from build123d import *

# Parameters (mm, degrees)
SKETCH_CAMERA_SEAT_W     = 16
SKETCH_CAMERA_SEAT_H     = 38
CAMERA_SEAT_DEPTH        = 3
FRONT_LIP_START          = 3
SKETCH_FRONT_LIP_W       = 16
SKETCH_FRONT_LIP_H       = 2.3
FRONT_LIP_DEPTH          = 7
REAR_LIP_START           = 3
SKETCH_REAR_LIP_W        = 16
SKETCH_REAR_LIP_H        = 2.3
REAR_LIP_DEPTH           = 4
STRAP_SLOTS_START        = -1
SKETCH_STRAP_SLOTS_W     = 8
SKETCH_STRAP_SLOTS_H     = 2.5
STRAP_SLOTS_DEPTH        = 5
M3_THROUGH_START         = -1
SKETCH_M3_THROUGH_R      = 1.7
M3_THROUGH_DEPTH         = 5
FLAT_HEAD_90DEG_START    = 1.5
SKETCH_FLAT_HEAD_90DEG_R = 1.5
FLAT_HEAD_90DEG_DEPTH    = 1.5
FLAT_HEAD_90DEG_TAPER    = -45


with BuildPart() as part:
    # Sketch_Camera_seat → Camera_seat (new body)
    with BuildSketch(Plane.XY):
        Rectangle(SKETCH_CAMERA_SEAT_W, SKETCH_CAMERA_SEAT_H)
    extrude(amount=CAMERA_SEAT_DEPTH)

    # Sketch_Front_lip → Front_lip (add)
    with BuildSketch(Plane.XY.offset(FRONT_LIP_START)):
        with Locations((0, -18.8)):
            Rectangle(SKETCH_FRONT_LIP_W, SKETCH_FRONT_LIP_H)
    extrude(amount=FRONT_LIP_DEPTH)

    # Sketch_Rear_lip → Rear_lip (add)
    with BuildSketch(Plane.XY.offset(REAR_LIP_START)):
        with Locations((0, 18.8)):
            Rectangle(SKETCH_REAR_LIP_W, SKETCH_REAR_LIP_H)
    extrude(amount=REAR_LIP_DEPTH)

    # Sketch_Strap_slots → Strap_slots (cut)
    with BuildSketch(Plane.XY.offset(STRAP_SLOTS_START)):
        with Locations((0, -10)):
            Rectangle(SKETCH_STRAP_SLOTS_W, SKETCH_STRAP_SLOTS_H)
        with Locations((0, 10)):
            Rectangle(SKETCH_STRAP_SLOTS_W, SKETCH_STRAP_SLOTS_H)
    extrude(amount=STRAP_SLOTS_DEPTH, mode=Mode.SUBTRACT)

    # Sketch_M3_through → M3_through (cut)
    with BuildSketch(Plane.XY.offset(M3_THROUGH_START)):
        with Locations((0, -15.5)):
            Circle(SKETCH_M3_THROUGH_R)
        with Locations((0, 15.5)):
            Circle(SKETCH_M3_THROUGH_R)
    extrude(amount=M3_THROUGH_DEPTH, mode=Mode.SUBTRACT)

    # Sketch_Flat_head_90deg → Flat_head_90deg (cut)
    with BuildSketch(Plane.XY.offset(FLAT_HEAD_90DEG_START)):
        with Locations((0, -15.5)):
            Circle(SKETCH_FLAT_HEAD_90DEG_R)
        with Locations((0, 15.5)):
            Circle(SKETCH_FLAT_HEAD_90DEG_R)
    extrude(amount=FLAT_HEAD_90DEG_DEPTH, taper=FLAT_HEAD_90DEG_TAPER, mode=Mode.SUBTRACT)


solid = part.part
Input: part model. Units: mm. Frame: model coordinates. A direction names the side the tool comes from. Give positions to 0.01 mm unless a question says otherwise; leave off trailing zeros. Write each loop counter-clockwise with the first axis right and the second up, starting at its lowest first coordinate (ties: lowest second). Pieces come first, ordered by that corner, then holes. Notation, with made-up numbers: M 21.25,73 L 41.25,73 A22 ccw 41.25,79 Z; hole C 72,-5 d7. An arc over 180 degrees is marked long. Use one line per item in the form item = value.
1. Mould query, pull axis Y, two halves, no side actions, for faces 4 (the face through (0, -19, 1)), 5 (the face through (0, -18, 3)), 6 (the face through (0, 19, 1)). Classes: released by +Y, released by -Y, zero draft, split by the parting line, or undercut.
Outcome:
face_4 = released by -Y
face_5 = undercut
face_6 = released by +Y
2. Cut plane D-D on x = 0. State how many separate pieces and enclosed holes the cut face has, and give its area (3 significant figures).
Outcome:
separate_pieces = 5
enclosed_holes = 0
area = 101 mm²
3. First-contact query: P1, Ø3.5, axis at x = -2, z = 1, coming from the +Y side; P2, Ø1.5, axis at x = -1.5, z = 2, coming from the -Y side; P3, Ø0.5, axis at x = 1, y = -19.5, coming from the -Z side; P4, Ø2, axis at x = 0, y = -15.5, coming from the +Z side. Flat tips, straight axial feed; report the tip coordinate or a pass-through.
Outcome:
P1 = 19
P2 = -19
P3 = 3
P4 = through
4. Cut plane B-B on z = 4.75. Return loops of the section in (x, y), and give its area (3 significant figures).
Outcome:
outline = M -8,-19.95 L 8,-19.95 L 8,-17.65 L -8,-17.65 Z; M -8,17.65 L 8,17.65 L 8,19.95 L -8,19.95 Z
area = 73.6 mm²
5. Cut plane C-C on y = 9.5. Return loops of the section in (x, z).
Outcome:
outline = M -8,0 L -4,0 L -4,3 L -8,3 Z; M 4,0 L 8,0 L 8,3 L 4,3 Z
6. Ray query, L1, parallel to Y at x = 0, z = 0.8; L2, parallel to Y at x = 1, z = 3.75; L3, parallel to Y at x = 0.75, z = 1.5. Return the intervals inside material, ascending.
Outcome:
L1 = -19 to -17.2, -13.8 to -11.25, -8.75 to 8.75, 11.25 to 13.8, 17.2 to 19
L2 = -19.95 to -17.65, 17.65 to 19.95
L3 = -19 to -17.03, -13.97 to -11.25, -8.75 to 8.75, 11.25 to 13.97, 17.03 to 19
7. Cut plane A-A on x = 3.5. Return loops of the section in (y, z).
Outcome:
outline = M -19.95,3 L -19,3 L -19,0 L -11.25,0 L -11.25,3 L -17.65,3 L -17.65,10 L -19.95,10 Z; M -8.75,0 L 8.75,0 L 8.75,3 L -8.75,3 Z; M 11.25,0 L 19,0 L 19,3 L 19.95,3 L 19.95,7 L 17.65,7 L 17.65,3 L 11.25,3 Z
8. Reachability of faces 1 (the face through (-0.1, -19.5, 3)), 2 (the face through (0, -17.65, 6)), 3 (the face through (0, 11.25, 1)) from +Z, -Z, +X, -X, +Y, -Y: full face, straight path, thin tool, end or side. Return the list, or none.
Outcome:
face_1 = -Z, +X, -X, -Y
face_2 = +Z, +X, -X
face_3 = +Z, -Z
